Here's how the part is built. I have some questions about the finished solid (model axes, mm). A direction names the side the tool comes from. Round coordinates to 2 decimals unless told otherwise and drop trailing zeros. Order: outer loops, then holes, each group sorted by start corner. A loop starts at its lowest first (then second) coordinate and runs counter-clockwise, first axis right, second up.
```python
from build123d import *

# Parameters (mm, degrees)
F0_W     = 400
F0_H     = 100
F1_DEPTH = 100
F2_W     = 50
F2_H     = 50
F3_DEPTH = 100
F4_W     = 50
F4_H     = 400
F5_DEPTH = 20


with BuildPart() as f1:
    # F0 (on Right) → F1 (new body)
    with BuildSketch(Plane.YZ):
        with Locations((-6.60181, 8.23221)):
            Rectangle(F0_W, F0_H)
    extrude(amount=F1_DEPTH)

    # F2 (on face) → F3 (cut)
    with BuildSketch(Plane.YZ.offset(100)):
        with Locations((-181.60181, 8.23221)):
            Rectangle(F2_W, F2_H)
    extrude(amount=-F3_DEPTH, mode=Mode.SUBTRACT)

    # F4 (on face) → F5 (join)
    with BuildSketch(Plane.XY.offset(58.23221)):
        with Locations((50, -6.60181)):
            Rectangle(F4_W, F4_H)
    extrude(amount=F5_DEPTH)


solid = f1.part
```
1. I need wall thicknesses on probe 1 along Z at (x, y) = (28, -157); probe 2 along Z at (x, y) = (5.5, -50); probe 3 along Y at (x, z) = (54.5, 14.5). Which ranges of each line are inside material? Lowest first, please.
Evaluation:
probe 1: z = -41.77 to -16.77, 33.23 to 78.23
probe 2: z = -41.77 to 58.23
probe 3: y = -156.6 to 193.4
2. On a 3-axis mill with a long thin cutter (end or side, diameter ignored), from which of +Z, -Z, +X, -X, +Y, -Y can I reach the whole of each face in a straight line? I mean faces 1 (the flat face through (25, -9, 68)), 2 (the flat face through (50, -4, 78.232)), 3 (the flat face through (87, -9, 58.232)), 4 (the flat face through (51, -182, 33.232)). Say none if no direction works.
Evaluation:
face 1: +Z, -X, +Y, -Y
face 2: +Z, +X, -X, +Y, -Y
face 3: +Z, +X, +Y, -Y
face 4: +X, -X, -Y
3. If we section it at A-A, the plane y = -177.5: Write out the boundary of the cut face in (x, z), and give its area (3 significant figures).
Evaluation:
outline: (0, -41.77) - (100, -41.77) - (100, -16.77) - (0, -16.77) - close; (0, 33.23) - (100, 33.23) - (100, 58.23) - (75, 58.23) - (75, 78.23) - (25, 78.23) - (25, 58.23) - (0, 58.23) - close
area: 6,000 mm2
4. If we section it at D-D, the plane z = 18.5: Write out the boundary of the cut face in (x, y).
Evaluation:
outline: (0, -156.6) - (100, -156.6) - (100, 193.4) - (0, 193.4) - close
5. I'm going to push flat-ended pins straight in: P1, Ø6, axis at x = 59.5, z = 24, coming from the -Y side; P2, Ø20, axis at x = 88, y = -63, coming from the +Z side; P3, Ø10, axis at y = 69, z = 72.5, coming from the +X side. Where does each tip first touch, or does it pass through?
Evaluation:
P1: stops at y = -156.6
P2: stops at z = 58.23
P3: stops at x = 75
6. If we section it at C-C, the plane y = 60.5: Write out the boundary of the cut face in (x, z).
Evaluation:
outline: (0, -41.77) - (100, -41.77) - (100, 58.23) - (75, 58.23) - (75, 78.23) - (25, 78.23) - (25, 58.23) - (0, 58.23) - close
7. If we section it at B-B, the plane x = 15.5: Write out the boundary of the cut face in (y, z), and give its area (3 significant figures).
Evaluation:
outline: (-206.6, -41.77) - (193.4, -41.77) - (193.4, 58.23) - (-206.6, 58.23) - (-206.6, 33.23) - (-156.6, 33.23) - (-156.6, -16.77) - (-206.6, -16.77) - close
area: 37,500 mm2
8. If we mould it in two halves opening along Z, with no side actions, what happens to faces 5 (the flat face through (51, -156.602, 8)), 6 (the flat face through (12, -9, 58.232)), 7 (the flat face through (0, -9, 9))? For each: released by +Z, released by -Z, zero draft, split by the parting line, or undercut.
Evaluation:
face 5: undercut
face 6: released by +Z
face 7: zero draft
